from build123d import *

# Parameters (mm, degrees)
SKETCH055_W          = 10
SKETCH055_H          = 121
SKETCH055_R          = 1.75
PAD026_DEPTH         = 5
SKETCH056_R          = 2.6
POCKET026_DEPTH      = 0.001
POCKET026_DEPTH_BACK = 542.783232
CHAMFER002_SIZE      = 1.75


with BuildPart() as part:
    # Sketch055 → Pad026 (new body)
    with BuildSketch(Plane.XY):
        with Locations((537.782232, -339.706519)):
            Rectangle(SKETCH055_W, SKETCH055_H)
        with Locations((537.782232, -381.20917)):
            Circle(SKETCH055_R, mode=Mode.SUBTRACT)
        with Locations((537.782232, -284.706588)):
            Circle(SKETCH055_R, mode=Mode.SUBTRACT)
    extrude(amount=PAD026_DEPTH)

    # Sketch056 → Pocket026 (cut, two sides)
    with BuildSketch(Plane.YZ) as pocket026_sk:
        with Locations((-392.25561, 5)):
            Circle(SKETCH056_R)
        with BuildLine():
            ThreePointArc((-357.457814, 7.6), (-360.057814, 5), (-357.457814, 2.4))
            Line((-357.457814, 2.4), (-296.002518, 2.4))
            ThreePointArc((-296.002518, 2.4), (-293.402518, 5), (-296.002518, 7.6))
            Line((-357.457814, 7.6), (-296.002518, 7.6))
        make_face()
    extrude(amount=-POCKET026_DEPTH, mode=Mode.SUBTRACT)
    extrude(pocket026_sk.sketch, amount=POCKET026_DEPTH_BACK, mode=Mode.SUBTRACT)

    # Chamfer002
    chamfer002_edges = [part.edges().sort_by_distance(p)[0] for p in [
        (536.032232, -381.20917, 0),
        (536.032232, -284.706588, 0),
    ]]
    chamfer(chamfer002_edges, length=CHAMFER002_SIZE)


solid = part.part
The model under review builds one solid part; all positions refer to its coordinate system, in mm. A direction names the side the tool comes from. Coordinates: 2 decimals unless noted, no trailing zeros. Order: outer loops, then holes, each group sorted by start corner. A loop starts at its lowest first (then second) coordinate and runs counter-clockwise, first axis right, second up. Notation, with made-up numbers: (55.5, 65) -> (83.5, 65) arc R19 cw to (83.5, 101) -> close; hole circle Ø7 at (47.5, 74.5). An arc over 180 degrees is marked (long way). Answer in a Markdown table with one row per item.
(1) Insertion check: pin 1 (1.5 mm diameter, centred on x = 541, y = -307.5, fed in from +Z). The pin has a flat end and moves straight along its axis. Give the tip position at first contact, or say it passes through.
Answers:
| item | result |
|---|---|
| pin 1 | z = 2.4 |
(2) The part is to be moulded in two halves that separate along Y. For faces 3 (the flat face through (538, -397, 5)), 4 (the flat face through (538, -279.207, 2)), 5 (the flat face through (538, -327, 2.4)), say which applies: +Y half, -Y half, draft (parallel to the pull), parting line (faces both ways), or undercut.
Answers:
| item | result |
|---|---|
| face 3 | draft |
| face 4 | +Y half |
| face 5 | undercut |
(3) Wall thickness on line 1 along Y through (x, z) = (535.5, 3); line 2 along Y through (x, z) = (536.75, 3.45); line 3 along Y through (x, z) = (540.75, 3.4) (3 decimals): over which ranges is each line inside the solid? List them lowest first.
Answers:
| item | result |
|---|---|
| line 1 | -400.21 to -393.92, -390.59 to -359.12, -294.34 to -279.21 |
| line 2 | -400.21 to -394.34, -390.17 to -382.62, -379.8 to -359.55, -293.92 to -286.12, -283.29 to -279.21 |
| line 3 | -400.207 to -394.305, -390.206 to -359.507, -293.953 to -279.207 |
(4) Consider section B-B (y = -391). Write out the cut boundary in (x, z).
Answers:
| item | result |
|---|---|
| outline | (532.78, 0) -> (542.78, 0) -> (542.78, 2.72) -> (532.78, 2.72) -> close |
(5) Consider section A-A (y = -353). Write out the cut boundary in (x, z).
Answers:
| item | result |
|---|---|
| outline | (532.78, 0) -> (542.78, 0) -> (542.78, 2.4) -> (532.78, 2.4) -> close |
(6) Machinability: for faces 1 (the flat face through (538, -339, 0)), 2 (the cylindrical face through (537.712, -294.184, 3.141)), which of the approach directions +Z, -Z, +X, -X, +Y, -Y give a long, thin tool a straight path to every point of the face, cutting with its end or side? Answer none if there is none.
Answers:
| item | result |
|---|---|
| face 1 | -Z, +X, -X, +Y, -Y |
| face 2 | +Z, +X, -X |
